```python
from build123d import *

# Parameters (mm, degrees)
SKETCH1_W           = 37
SKETCH1_H           = 21.6
BOSS_EXTRUDE1_DEPTH = 2
SKETCH2_W           = 6
SKETCH2_H           = 1.5
SKETCH2_W_2         = 1.5
SKETCH2_H_2         = 5
BOSS_EXTRUDE2_DEPTH = 22.44
SKETCH3_W           = 6
SKETCH3_H           = 3
BOSS_EXTRUDE3_DEPTH = 5
CHAMFER1_SIZE       = 5
SKETCH4_W           = 6
SKETCH4_H           = 3
BOSS_EXTRUDE4_DEPTH = 5
CHAMFER2_SIZE       = 5
SKETCH6_W           = 5
SKETCH6_H           = 7.52
SKETCH6_W_2         = 2.8
SKETCH6_H_2         = 5
CUT_EXTRUDE1_DEPTH  = 5
SKETCH8_W           = 20.25
SKETCH8_H           = 8.3
SKETCH8_W_2         = 10.75
SKETCH8_H_2         = 21.6
CUT_EXTRUDE3_DEPTH  = 10
FILLET1_R           = 1
FILLET2_R           = 1
SKETCH9_R           = 2
CUT_EXTRUDE4_DEPTH  = 10
SKETCH13_W          = 25
SKETCH13_H          = 7.533980582
BOSS_EXTRUDE5_DEPTH = 13.38
SKETCH14_R          = 2.4
CUT_EXTRUDE5_DEPTH  = 7.92
SKETCH15_R          = 3.1
SKETCH15_W          = 0.016515358
SKETCH15_H          = 0.077878544
CUT_EXTRUDE6_DEPTH  = 0.8
CUT_EXTRUDE7_START  = -0.8
SKETCH16_R          = 3.1
CUT_EXTRUDE7_DEPTH  = 0.8
SKETCH19_W          = 18.75
SKETCH19_H          = 6
CUT_EXTRUDE8_DEPTH  = 10
FILLET3_R           = 3.69
CHAMFER3_SIZE       = 1
CHAMFER4_SIZE       = 1


# Some blends are built 0.0001 mm under size
with BuildPart() as part:
    # Sketch1 → Boss-Extrude1 (new body)
    with BuildSketch(Plane(origin=(0, 0, 0), x_dir=(1, 0, 0), z_dir=(0, 1, 0))):
        Rectangle(SKETCH1_W, SKETCH1_H)
    extrude(amount=BOSS_EXTRUDE1_DEPTH)

    # Sketch2 → Boss-Extrude2 (add)
    with BuildSketch(Plane(origin=(0, 2, 0), x_dir=(1, 0, 0), z_dir=(0, 1, 0))):
        with Locations((-4.75, 10.05)):
            Rectangle(SKETCH2_W, SKETCH2_H)
        with Locations((-4.75, -10.05)):
            Rectangle(SKETCH2_W, SKETCH2_H)
        with Locations((17.75, 0)):
            Rectangle(SKETCH2_W_2, SKETCH2_H_2)
    extrude(amount=BOSS_EXTRUDE2_DEPTH)

    # Sketch3 → Boss-Extrude3 (add)
    with BuildSketch(Plane(origin=(0, 24.44, 0), x_dir=(1, 0, 0), z_dir=(0, 1, 0))):
        with Locations((-4.75, 9.3)):
            Rectangle(SKETCH3_W, SKETCH3_H)
    extrude(amount=BOSS_EXTRUDE3_DEPTH)

    # Chamfer1
    # the kernel refuses this chamfer: 5 mm, written as the material it takes off along each edge
    with BuildSketch(Plane(origin=(11.10841494, 29.44, -7.8), x_dir=(0, -0.9996219169112968, 0.027495876610586317), z_dir=(-1, 0, 0))) as chamfer1_piece_1:
        Polygon((CHAMFER1_SIZE * 0.999621916911, -CHAMFER1_SIZE * 0.0274958766106), (-CHAMFER1_SIZE * 0.0274958766106, -CHAMFER1_SIZE * 0.999621916911), (0, 0), align=None)
    extrude(amount=31.71682988, mode=Mode.SUBTRACT)

    # Sketch4 → Boss-Extrude4 (add)
    with BuildSketch(Plane(origin=(0, 24.44, 0), x_dir=(1, 0, 0), z_dir=(0, 1, 0))):
        with Locations((-4.75, -9.3)):
            Rectangle(SKETCH4_W, SKETCH4_H)
    extrude(amount=BOSS_EXTRUDE4_DEPTH)

    # Chamfer2
    # the kernel refuses this chamfer: 5 mm, written as the material it takes off along each edge
    with BuildSketch(Plane(origin=(11.10841494, 29.44, 7.8), x_dir=(0, -0.9996219169112968, -0.027495876610586317), z_dir=(-1, 0, 0))) as chamfer2_piece_1:
        Polygon((CHAMFER2_SIZE * 0.999621916911, CHAMFER2_SIZE * 0.0274958766106), (-CHAMFER2_SIZE * 0.0274958766106, CHAMFER2_SIZE * 0.999621916911), (0, 0), align=None)
    extrude(amount=31.71682988, mode=Mode.SUBTRACT)

    # Sketch6 → Cut-Extrude1 (cut)
    with BuildSketch(Plane(origin=(18.5, 0, 0), x_dir=(0, 0, -1), z_dir=(1, 0, 0))):
        with Locations((0, 20.68)):
            Rectangle(SKETCH6_W, SKETCH6_H)
        with Locations((0, 13.22)):
            Rectangle(SKETCH6_W_2, SKETCH6_H_2)
    extrude(amount=-CUT_EXTRUDE1_DEPTH, mode=Mode.SUBTRACT)

    # Sketch8 → Cut-Extrude3 (cut)
    with BuildSketch(Plane(origin=(0, 2, 0), x_dir=(1, 0, 0), z_dir=(0, 1, 0))):
        with Locations((8.375, 6.65)):
            Rectangle(SKETCH8_W, SKETCH8_H)
        with Locations((8.375, -6.65)):
            Rectangle(SKETCH8_W, SKETCH8_H)
        with Locations((-13.125, 0)):
            Rectangle(SKETCH8_W_2, SKETCH8_H_2)
    extrude(amount=-CUT_EXTRUDE3_DEPTH, mode=Mode.SUBTRACT)

    # Fillet1
    fillet1_edges = [part.edges().sort_by_distance(p)[0] for p in [
        (-4.75, 0, -10.8),
        (18.5, 0, 0),
        (-4.75, 0, 10.8),
        (-4.75, 27.44, -10.8),
        (-4.75, 27.44, 10.8),
    ]]
    fillet(fillet1_edges, radius=FILLET1_R)

    # Fillet2
    fillet2_edges = [part.edges().sort_by_distance(p)[0] for p in [
        (18.5, 16.92, 0),
    ]]
    fillet(fillet2_edges, radius=FILLET2_R)

    # Sketch9 → Cut-Extrude4 (cut)
    with BuildSketch(Plane.XY.offset(-9.3)):
        with Locations((-4.75, 13.22)):
            Circle(SKETCH9_R)
    extrude(amount=-CUT_EXTRUDE4_DEPTH, mode=Mode.SUBTRACT)

    # Sketch13 → Boss-Extrude5 (add)
    with BuildSketch(Plane.XZ):
        with Locations((4.75, 0)):
            Rectangle(SKETCH13_W, SKETCH13_H)
    extrude(amount=BOSS_EXTRUDE5_DEPTH)

    # Sketch14 → Cut-Extrude5 (cut)
    with BuildSketch(Plane.XY.offset(3.766990291)):
        with Locations((4.75, -9.69)):
            Circle(SKETCH14_R)
        with Locations((12.72, -9.69)):
            Circle(SKETCH14_R)
        with Locations((-3.22, -9.69)):
            Circle(SKETCH14_R)
    extrude(amount=-CUT_EXTRUDE5_DEPTH, mode=Mode.SUBTRACT)

    # Sketch15 → Cut-Extrude6 (cut)
    with BuildSketch(Plane.XY.offset(3.766990291)):
        with Locations((-3.22, -9.69)):
            Circle(SKETCH15_R)
        with Locations((4.75, -9.69)):
            Circle(SKETCH15_R)
        with Locations((12.72, -9.69)):
            Circle(SKETCH15_R)
        with Locations((1.021954756, -12.130200689)):
            Rectangle(SKETCH15_W, SKETCH15_H)
    extrude(amount=-CUT_EXTRUDE6_DEPTH, mode=Mode.SUBTRACT)

    # Sketch16 → Cut-Extrude7 (cut)
    with BuildSketch(Plane(origin=(0, 0, -3.766990291), x_dir=(-1, 0, 0), z_dir=(0, 0, -1)).offset(CUT_EXTRUDE7_START)):
        with Locations(Location((-4.75, -9.69, 0), (0, 0, 180))):
            Circle(SKETCH16_R)
        with Locations(Location((3.22, -9.69, 0), (0, 0, 180))):
            Circle(SKETCH16_R)
        with Locations(Location((-12.72, -9.69, 0), (0, 0, 180))):
            Circle(SKETCH16_R)
    extrude(amount=CUT_EXTRUDE7_DEPTH, mode=Mode.SUBTRACT)

    # Sketch19 → Cut-Extrude8 (cut)
    with BuildSketch(Plane(origin=(0, 0, -3.766990291), x_dir=(-1, 0, 0), z_dir=(0, 0, -1))):
        with Locations((-7.875, -3)):
            Rectangle(SKETCH19_W, SKETCH19_H)
    extrude(amount=-CUT_EXTRUDE8_DEPTH, mode=Mode.SUBTRACT)

    # Fillet3
    fillet3_edges = [part.edges().sort_by_distance(p)[0] for p in [
        (-7.75, -13.38, 0),
        (17.25, -13.38, 0),
        (17.25, -6, 0),
    ]]
    fillet(fillet3_edges, radius=FILLET3_R - 0.0001)  # a hair under: the kernel refuses the full size

    # Chamfer3
    # the kernel refuses this chamfer: 1 mm, written as the material it takes off along each edge
    with BuildSketch(Plane(origin=(-1.5, 0, -6.338673279), x_dir=(0.027495876610586275, -0.9996219169112968, 0), z_dir=(0, 0, 1))) as chamfer3_piece_1_section:
        Polygon((CHAMFER3_SIZE * 0.999621916911, -CHAMFER3_SIZE * 0.0274958766106), (-CHAMFER3_SIZE * 0.0274958766106, -CHAMFER3_SIZE * 0.999621916911), (0, 0), align=None)
    chamfer3_piece_1 = extrude(amount=3.838673279, mode=Mode.PRIVATE)
    chamfer3_piece_1 = split(chamfer3_piece_1, bisect_by=Plane(origin=(-1.75, -0.44047619, -3.133495146), z_dir=(1, 0, 0)), keep=Keep.TOP, mode=Mode.PRIVATE)
    add(chamfer3_piece_1, mode=Mode.SUBTRACT)

    # Chamfer4
    # the kernel refuses this chamfer: 1 mm, written as the material it takes off along each edge
    with BuildSketch(Plane(origin=(-1.5, 0, 2.5), x_dir=(-0.9996219169112968, 0.027495876610586358, 0), z_dir=(0, 0, 1))) as chamfer4_piece_1_section:
        Polygon((CHAMFER4_SIZE * 0.999621916911, CHAMFER4_SIZE * 0.0274958766106), (-CHAMFER4_SIZE * 0.0274958766106, CHAMFER4_SIZE * 0.999621916911), (0, 0), align=None)
    chamfer4_piece_1 = extrude(amount=3.838673279, mode=Mode.PRIVATE)
    chamfer4_piece_1 = split(chamfer4_piece_1, bisect_by=Plane(origin=(-1.75, -0.44047619, 3.133495146), z_dir=(1, 0, 0)), keep=Keep.TOP, mode=Mode.PRIVATE)
    add(chamfer4_piece_1, mode=Mode.SUBTRACT)


solid = part.part
```
Input: part model. Units: mm. Frame: model coordinates. A direction names the side the tool comes from. Give positions to 0.01 mm unless a question says otherwise; leave off trailing zeros. Order: outer loops, then holes, each group sorted by start corner. A loop starts at its lowest first (then second) coordinate and runs counter-clockwise, first axis right, second up. Notation, with made-up numbers: (66, 82.5) - (122, 82.5) arc R26 cw to (122, 98.5) - close; hole circle Ø1 at (-13, 52). An arc over 180 degrees is marked (long way). One line per item, written item: value.
1. Cut plane D-D, the plane z = 4.5. Output: boundary loops of the cut face in (x, y).
Determined:
outline: (-7.75, 0) - (-1.75, 0) - (-1.75, 2) - (-7.75, 2) - close
2. Reachability of faces 1 (the face through (18, 13, 1.4)), 2 (the face through (-4.71, 25.08, -8.44)), 3 (the face through (-1.79, -6.94, -3.36)), 4 (the face through (14.937, -10.609, 0.042)), 5 (the face through (4.078, -12.716, 3.373)) from +Z, -Z, +X, -X, +Y, -Y: full face, straight path, thin tool, end or side. Return the list, or none.
Determined:
face 1: +X, -X
face 2: +X, -X, +Y
face 3: -Z
face 4: +Z, -Z
face 5: +Z
3. Draft query along X for faces 6 (the face through (18, 13, -1.4)), 7 (the face through (-0.93, -8.97, 0.04)), 8 (the face through (16.14, -7.05, 0.05)). Return one class per face: released by +X, released by -X, zero draft, split by the parting line, or undercut.
Determined:
face 6: zero draft
face 7: undercut
face 8: released by +X
4. Pin query (flat end, axial travel): pin 1 Ø10 at (y, z) = (-6, 7.5) entering from +X; pin 2 Ø1.5 at (y, z) = (3.5, -8.5) entering from +X; pin 3 Ø1.6 at (x, y) = (17.5, 14.5) entering from +Z; pin 4 Ø1.8 at (x, z) = (-3.5, 7.5) entering from -Y. Return the tip coordinate at first contact, or that it passes through.
Determined:
pin 1: x = 17.23
pin 2: through
pin 3: z = 2.5
pin 4: y = 0
5. Line query: probe 1 along Y at (x, z) = (4.75, -1); probe 2 along X at (y, z) = (-9.69, -3.5); probe 3 along X at (y, z) = (-9, -3). Output: solid intervals per line, ascending.
Determined:
probe 1: -13.38 to -12.09, -7.29 to -6, 0 to 2
probe 2: -7.75 to -6.32, -0.12 to 1.65, 7.85 to 9.62, 15.82 to 17.25
probe 3: -7.75 to -6.24, -0.2 to 1.73, 7.77 to 9.7, 15.74 to 17.18
6. Cut plane C-C, the plane y = 13.22. Output: boundary loops of the cut face in (x, z).
Determined:
outline: (-7.75, -10.8) - (-6.75, -10.8) - (-6.75, -9.3) - (-7.75, -9.3) - close; (-7.75, 9.3) - (-1.75, 9.3) - (-1.75, 10.8) - (-7.75, 10.8) - close; (-2.75, -10.8) - (-1.75, -10.8) - (-1.75, -9.3) - (-2.75, -9.3) - close; (17, -2.5) - (18.5, -2.5) - (18.5, -1.4) - (17, -1.4) - close; (17, 1.4) - (18.5, 1.4) - (18.5, 2.5) - (17, 2.5) - close
7. Cut plane A-A, the plane x = 4.75. Output: boundary loops of the cut face in (y, z).
Determined:
outline: (-13.38, -3.77) - (-12.79, -3.77) - (-12.79, -2.97) - (-12.09, -2.97) - (-12.09, 2.97) - (-12.79, 2.97) - (-12.79, 3.77) - (-13.38, 3.77) - close; (-7.29, -2.97) - (-6.59, -2.97) - (-6.59, -3.77) - (-6, -3.77) - (-6, 3.77) - (-6.59, 3.77) - (-6.59, 2.97) - (-7.29, 2.97) - close; (0, -2.5) - (2, -2.5) - (2, 2.5) - (0, 2.5) - close
8. Cut plane B-B, the plane y = 8.5. Output: boundary loops of the cut face in (x, z), and give its area (3 significant figures).
Determined:
outline: (-7.75, -10.8) - (-1.75, -10.8) - (-1.75, -9.3) - (-7.75, -9.3) - close; (-7.75, 9.3) - (-1.75, 9.3) - (-1.75, 10.8) - (-7.75, 10.8) - close; (17, -2.5) - (18.5, -2.5) - (18.5, 2.5) - (17, 2.5) - close
area: 25.5 mm2
